The listing builds one solid part. Answer for the finished solid, in the listing's coordinates (mm). Face numbers are marked on the shaded views. A direction names the side the tool comes from. Give positions to 0.01 mm unless a question says otherwise; leave off trailing zeros. Order: outer loops, then holes, each group sorted by start corner. A loop starts at its lowest first (then second) coordinate and runs counter-clockwise, first axis right, second up. Notation, with made-up numbers: (-16, 84) - (-7, 84) arc R11 ccw to (-7, 102) - close; hole circle Ø11 at (-4.5, 47). An arc over 180 degrees is marked (long way). Use a Markdown table: item, result. Add a question column.
1) The mould has two halves that part along Z. Classify the marked faces 3, 4 and 5: released by +Z, released by -Z, zero draft, split by the parting line, or undercut.
2) Straight lines are drawn through the part: line 1 (Z direction, x = -29.5, y = -122); line 2 (X direction, y = -9, z = -71); line 3 (Z direction, x = -55, y = -82). For each, find the intervals that lie inside material, in ascending order.
3) Find section A-A, the plane x = 73.5. Determine the outline of the cut face in (y, z).
4) A flat-ended cylindrical pin translates along its axis: pin 1 (3 mm diameter, centred on x = 68.5, z = -19.5, fed in from -Y). Find the tip coordinate at first contact, or state that the pin passes through.
5) For the marked faces 1 and 2, determine the directions among +Z, -Z, +X, -X, +Y, -Y from which every point of the face is accessible in a straight line to the end or side of a thin tool.
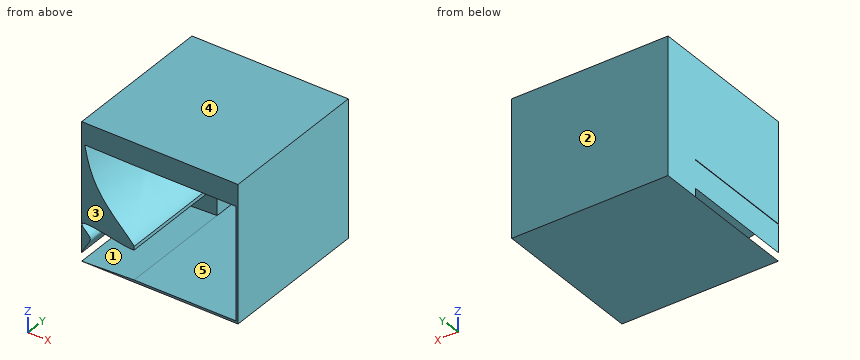
from build123d import *

# Parameters (mm, degrees)
F0_W      = 181.4180165529
F0_H      = 158.4694236517
F1_DEPTH  = 177.8
F2_T      = -2.54
F3_W      = 58.3408249235
F3_H      = 153.3894236517
F4_DEPTH  = 175.26
F5_W      = 117.9971916294
F5_H      = 23.1996511734
F6_DEPTH  = 175.26
F8_DEPTH  = 155.448
F9_DEPTH  = 21.59
F10_DEPTH = 21.59


with BuildPart() as f1:
    # F0 (on Front) → F1 (new body)
    with BuildSketch(Plane.XZ):
        Rectangle(F0_W, F0_H)
    extrude(amount=F1_DEPTH)

    # F2
    f2_openings = [f1.faces().sort_by_distance(p)[0] for p in [
        (0, -177.8, 0),
    ]]
    offset(amount=F2_T, openings=f2_openings)

    # F3 (on face) → F4 (join)
    with BuildSketch(Plane.XZ.offset(2.54)):
        with Locations((-58.9985958147, 0)):
            Rectangle(F3_W, F3_H)
    extrude(amount=F4_DEPTH)

    # F5 (on face) → F6 (join)
    with BuildSketch(Plane.XZ.offset(2.54)):
        with Locations((29.1704124618, 65.0948862392)):
            Rectangle(F5_W, F5_H)
    extrude(amount=F6_DEPTH)

    # F7 (on face) → F8 (cut)
    with BuildSketch(Plane.XZ.offset(177.8)):
        with BuildLine():
            Line((-29.8281833529, 53.4950606525), (-87.1266858607, 54.1800689548))
            add(Edge.make_bspline(
                [(-87.1266858607, 54.1800689548), (-84.1960310539, 37.7339910826), (-73.3918905439, 0.0733245961), (-35.1075253937, -30.5161568282), (-29.8281833529, -38.5061018169)],
                knots=[0.0711804972, 0.0711804972, 0.0711804972, 0.0711804972, 0.2125760889, 0.4036272484, 0.4036272484, 0.4036272484, 0.4036272484], degree=3))
            Line((-29.8281833529, -38.5061018169), (-29.8281833529, 53.4950606525))
        make_face()
        with BuildLine():
            Line((-29.8281833529, -76.6947118258), (-29.8281833529, -42.6409877837))
            add(Edge.make_bspline(
                [(-29.8281833529, -42.6409877837), (-35.4231693122, -44.7782083287), (-76.9735240129, -33.3987697863), (-96.3430681195, -35.7142988828), (-78.4077125974, -48.2869849637), (-82.5900483234, -55.7535374326), (-91.3199582214, -69.1015545227), (-90.8273371486, -70.6873939206), (-90.7090082765, -71.0683166981)],
                knots=[0.4534884255, 0.4534884255, 0.4534884255, 0.4534884255, 0.6260487265, 0.7112245832, 0.8039358777, 0.872883826, 0.969466362, 1, 1, 1, 1], degree=3))
            Line((-90.7090082765, -71.0683166981), (-90.7090082765, -79.2347118258))
            Line((-90.7090082765, -79.2347118258), (-29.8281833529, -76.6947118258))
        make_face()
        with BuildLine():
            add(Edge.make_bspline(
                [(-29.8281833529, -38.5061018169), (-28.4503628307, -40.5913446544), (-28.2115161111, -42.0234394165), (-29.8281833529, -42.6409877837)],
                knots=[0.4036272484, 0.4036272484, 0.4036272484, 0.4036272484, 0.4534884255, 0.4534884255, 0.4534884255, 0.4534884255], degree=3))
            Line((-29.8281833529, -38.5061018169), (-29.8281833529, -42.6409877837))
        make_face()
    extrude(amount=-F8_DEPTH, mode=Mode.SUBTRACT)

    # F9 (cut): a face of the model
    f9_faces = [f1.faces().sort_by_distance(p)[0] for p in [
        (-52.0616522206, -22.352, 20.2283924947),
    ]]
    extrude(f9_faces, amount=-F9_DEPTH, mode=Mode.SUBTRACT)

    # F10 (add): a face of the model
    f10_faces = [f1.faces().sort_by_distance(p)[0] for p in [
        (-59.9035044094, -22.352, -58.7218342299),
    ]]
    extrude(f10_faces, amount=F10_DEPTH)


solid = f1.part
The answers:
| question | item | result |
|---|---|---|
| 1 | face 3 | zero draft |
| 1 | face 4 | released by +Z |
| 1 | face 5 | undercut |
| 2 | line 1 | -79.23 to -76.69, 53.5 to 79.23 |
| 2 | line 2 | -90.71 to -29.83, 88.17 to 90.71 |
| 2 | line 3 | -79.23 to -77.74, -39.61 to -11.93, 53.8 to 79.23 |
| 3 | outline | (-177.8, -79.23) - (0, -79.23) - (0, 79.23) - (-177.8, 79.23) - (-177.8, 53.5) - (-2.54, 53.5) - (-2.54, -76.69) - (-177.8, -76.69) - close |
| 4 | pin 1 | y = -2.54 |
| 5 | face 1 | -X, -Y |
| 5 | face 2 | +Z, -Z, +X, -X, +Y |
